Geometry check sheet. Reference: drawing and pictorial views, mm from the part's lowest x, y, z. A direction names the side the tool comes from. Coordinates: 2 decimals unless noted, no trailing zeros. Loops run counter-clockwise (first coordinate to the right, second up) from the corner with the lowest first, then second, coordinate; pieces in that order, holes last. Notation, with made-up numbers: (-10.5, 20) -> (22.5, 20) arc R8 ccw to (22.5, 29) -> close; hole circle Ø11 at (-11.75, -37.75). An arc over 180 degrees is marked (long way). Answer as a JSON object with one key per item and string values.
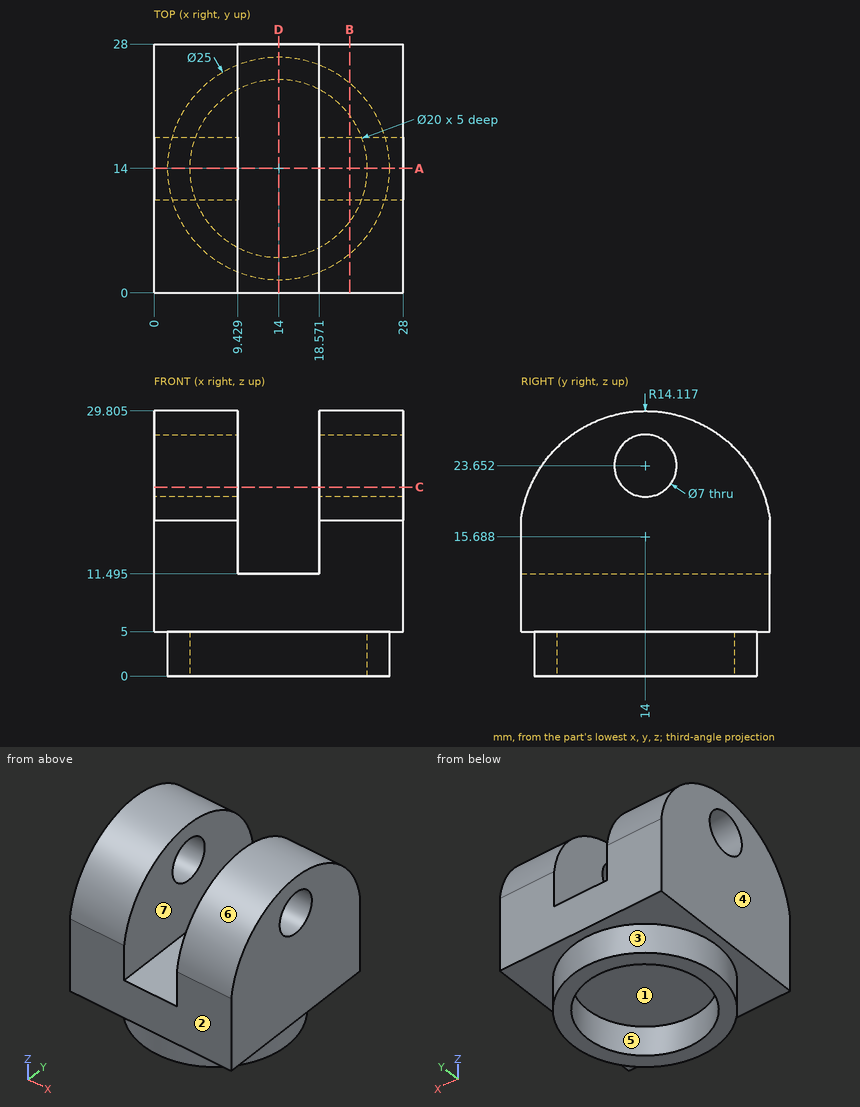
1. Mould release check, pull along X, two halves, no side actions. Record for the marked faces 1, 2, 3 and 4: released by +X, released by -X, zero draft, split by the parting line, or undercut.
Evaluation:
{"face 1": "undercut", "face 2": "zero draft", "face 3": "split by the parting line", "face 4": "released by -X"}
2. Tool access check on the marked faces 5, 6 and 7. Record the directions out of +Z, -Z, +X, -X, +Y, -Y that give a thin tool (end or side, any length) a straight path to the whole face; none if there is none.
Evaluation:
{"face 5": "-Z", "face 6": "+Z, +X, -X", "face 7": "+Z, +Y, -Y"}
3. Section check A-A, the plane y = 14. Record the boundary of the cut face in (x, z) (1 decimal).
Evaluation:
{"outline": "(0, 5) -> (1.5, 5) -> (1.5, 0) -> (4, 0) -> (4, 5) -> (24, 5) -> (24, 0) -> (26.5, 0) -> (26.5, 5) -> (28, 5) -> (28, 20.2) -> (18.6, 20.2) -> (18.6, 11.5) -> (9.4, 11.5) -> (9.4, 20.2) -> (0, 20.2) -> close; (0, 27.2) -> (9.4, 27.2) -> (9.4, 29.8) -> (0, 29.8) -> close; (18.6, 27.2) -> (28, 27.2) -> (28, 29.8) -> (18.6, 29.8) -> close"}
4. Section check D-D, the plane x = 14. Record the boundary of the cut face in (y, z) (1 decimal).
Evaluation:
{"outline": "(0, 5) -> (1.5, 5) -> (1.5, 0) -> (4, 0) -> (4, 5) -> (24, 5) -> (24, 0) -> (26.5, 0) -> (26.5, 5) -> (28, 5) -> (28, 11.5) -> (0, 11.5) -> close"}
5. Section check C-C, the plane z = 21.25. Record the boundary of the cut face in (x, y) (1 decimal), then the cut area to 3 significant figures.
Evaluation:
{"outline": "(0, 1) -> (9.4, 1) -> (9.4, 11.5) -> (0, 11.5) -> close; (0, 16.5) -> (9.4, 16.5) -> (9.4, 27) -> (0, 27) -> close; (18.6, 1) -> (28, 1) -> (28, 11.5) -> (18.6, 11.5) -> close; (18.6, 16.5) -> (28, 16.5) -> (28, 27) -> (18.6, 27) -> close", "area": "393 mm^2"}
6. Section check B-B, the plane x = 22. Record the boundary of the cut face in (y, z) (1 decimal).
Evaluation:
{"outline": "(0, 5) -> (4.4, 5) -> (4.4, 0) -> (8, 0) -> (8, 5) -> (20, 5) -> (20, 0) -> (23.6, 0) -> (23.6, 5) -> (28, 5) -> (28, 17.5) arc R14.1 ccw to (0, 17.5) -> close; hole circle Ø7 at (14, 23.7)"}
7. Depth check by flat-ended pin: P1, Ø6, axis at x = 13.5, y = 14, coming from the -Z side; P2, Ø2, axis at x = 23, y = 21, coming from the +Z side; P3, Ø5, axis at x = 17, z = 19.5, coming from the -Y side. Enter the tip coordinate at first touch or a pass-through.
Evaluation:
{"P1": "stops at z = 5", "P2": "stops at z = 28.47", "P3": "stops at y = 0.01"}
8. Thickness scan on probe 1 along X at (y, z) = (24.25, 16.75); probe 2 along Y at (x, z) = (14, 3.2); probe 3 along Z at (x, y) = (10, 8.75) (1 decimal). Record the ranges inside material, lowest first. Write a range as from..to.
Evaluation:
{"probe 1": "x = 0..9.43, 18.57..28", "probe 2": "y = 1.5..4, 24..26.5", "probe 3": "z = 5..11.5"}
